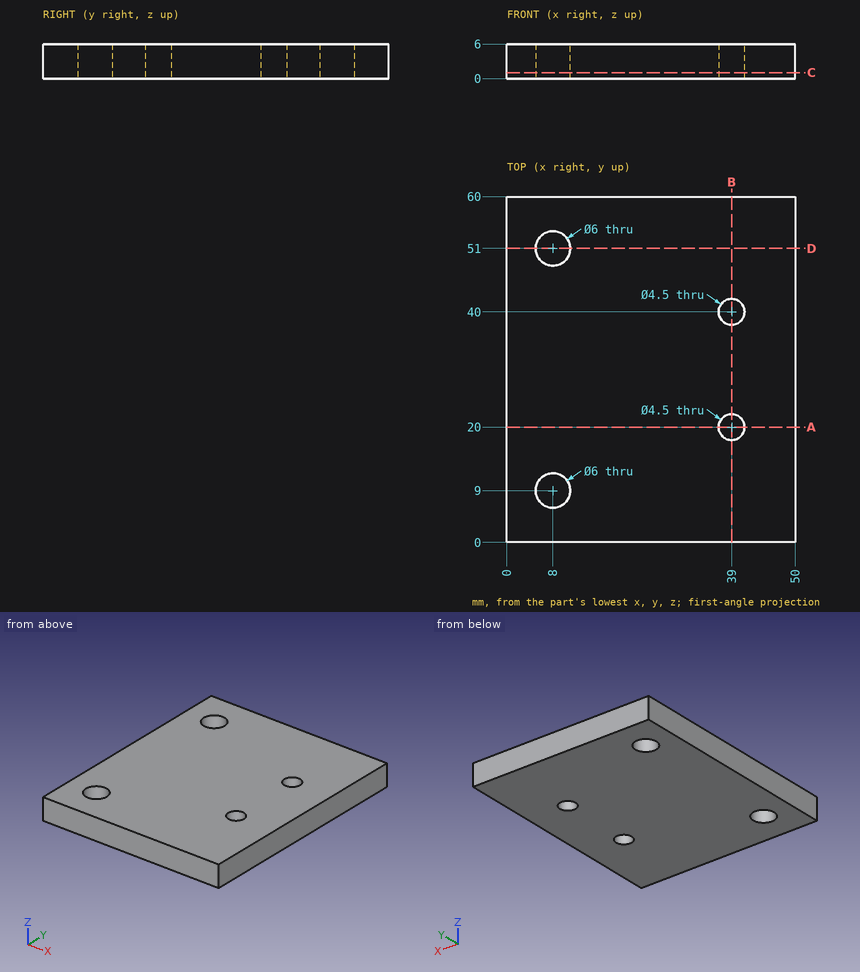
Source: three-view drawing plus pictorial views. Frame: mm from the lowest corner of the part. Coordinates: 2 decimals unless noted, no trailing zeros. Loops run counter-clockwise (first coordinate to the right, second up) from the corner with the lowest first, then second, coordinate; pieces in that order, holes last. Notation, with made-up numbers: (-14, 84) -> (25, 84) arc R28 ccw to (25, 123) -> close; hole circle Ø9 at (33.5, -5). An arc over 180 degrees is marked (long way). One line per item, written item: value.
(1) Pin query (flat end, axial travel): pin 1 Ø4 at (x, y) = (39, 20) entering from -Z. Return the tip coordinate at first contact, or that it passes through.
Answer below:
pin 1: passes through
(2) Cut plane C-C (z = 1.05). Output: boundary loops of the cut face in (x, y).
Answer below:
outline: (0, 0) -> (50, 0) -> (50, 60) -> (0, 60) -> close; hole circle Ø6 at (8, 9); hole circle Ø6 at (8, 51); hole circle Ø4.5 at (39, 20); hole circle Ø4.5 at (39, 40)
(3) Cut plane A-A (y = 20). Output: boundary loops of the cut face in (x, z).
Answer below:
outline: (0, 0) -> (36.75, 0) -> (36.75, 6) -> (0, 6) -> close; (41.25, 0) -> (50, 0) -> (50, 6) -> (41.25, 6) -> close
(4) Cut plane D-D (y = 51). Output: boundary loops of the cut face in (x, z), then the cut area to 3 significant figures.
Answer below:
outline: (0, 0) -> (5, 0) -> (5, 6) -> (0, 6) -> close; (11, 0) -> (50, 0) -> (50, 6) -> (11, 6) -> close
area: 264 mm2
(5) Ray query, line 1 along Y through (x, z) = (39, 2.35); line 2 along X through (y, z) = (40, 3.9); line 3 along X through (y, z) = (9, 1.45). Return the intervals inside material, ascending.
Answer below:
line 1: y = 0 to 17.75, 22.25 to 37.75, 42.25 to 60
line 2: x = 0 to 36.75, 41.25 to 50
line 3: x = 0 to 5, 11 to 50
(6) Cut plane B-B (x = 39). Output: boundary loops of the cut face in (y, z).
Answer below:
outline: (0, 0) -> (17.75, 0) -> (17.75, 6) -> (0, 6) -> close; (22.25, 0) -> (37.75, 0) -> (37.75, 6) -> (22.25, 6) -> close; (42.25, 0) -> (60, 0) -> (60, 6) -> (42.25, 6) -> close
